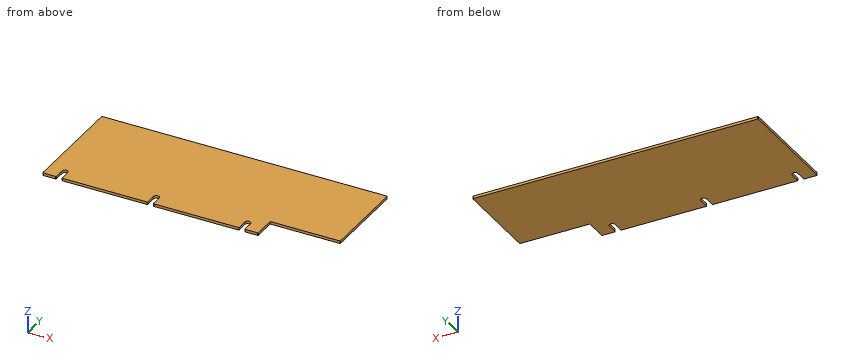
from build123d import *

# Parameters (mm, degrees)
PAD_DEPTH = 3


with BuildPart() as part:
    # Sketch → Pad (new body)
    with BuildSketch(Plane.XY):
        with BuildLine():
            Line((0, 126), (0, 1))
            ThreePointArc((0, 1), (0.292893, 0.292893), (1, 0))
            Line((1, 0), (14.748, 0))
            ThreePointArc((14.748, 0), (15.455107, 0.292893), (15.748, 1))
            Line((15.748, 12.7), (15.748, 1))
            ThreePointArc((22.352, 12.7), (19.05, 16.002), (15.748, 12.7))
            Line((22.352, 12.7), (22.352, 1))
            ThreePointArc((22.352, 1), (22.644893, 0.292893), (23.352, 0))
            Line((23.352, 0), (120.948, 0))
            ThreePointArc((120.948, 0), (121.655107, 0.292893), (121.948, 1))
            Line((121.948, 12.7), (121.948, 1))
            ThreePointArc((128.552, 12.7), (125.25, 16.002), (121.948, 12.7))
            Line((128.552, 12.7), (128.552, 1))
            ThreePointArc((128.552, 1), (128.844893, 0.292893), (129.552, 0))
            Line((129.552, 0), (227.148, 0))
            ThreePointArc((227.148, 0), (227.855107, 0.292893), (228.148, 1))
            Line((228.148, 12.7), (228.148, 1))
            ThreePointArc((234.752, 12.7), (231.45, 16.002), (228.148, 12.7))
            Line((234.752, 12.7), (234.752, 1))
            ThreePointArc((234.752, 1), (235.044893, 0.292893), (235.752, 0))
            Line((235.752, 0), (249.5, 0))
            ThreePointArc((249.5, 0), (250.207107, 0.292893), (250.5, 1))
            Line((250.5, 1), (250.5, 24.9))
            ThreePointArc((251.5, 25.9), (250.792893, 25.607107), (250.5, 24.9))
            Line((251.5, 25.9), (330.9999, 25.9))
            ThreePointArc((330.9999, 25.9), (331.707007, 26.192893), (331.9999, 26.9))
            Line((331.9999, 26.9), (331.9999, 126))
            ThreePointArc((331.9999, 126), (331.707007, 126.707107), (330.9999, 127))
            Line((330.9999, 127), (1, 127))
            ThreePointArc((1, 127), (0.292893, 126.707107), (0, 126))
        make_face()
    extrude(amount=PAD_DEPTH)


solid = part.part
Input: part model. Units: mm. Frame: model coordinates. Give positions to 0.01 mm unless a question says otherwise; leave off trailing zeros. Order: outer loops, then holes, each group sorted by start corner. A loop starts at its lowest first (then second) coordinate and runs counter-clockwise, first axis right, second up. Notation, with made-up numbers: (22.5, -25.75) - (62.5, -25.75) arc R9 cw to (62.5, -18.75) - close; hole circle Ø10 at (61, -17). An arc over 180 degrees is marked (long way). Answer as a JSON object with one key per item and string values. Group by question number.
Q1. Line query: probe 1 along X at (y, z) = (11.5, 2.6); probe 2 along Y at (x, z) = (297, 1); probe 3 along X at (y, z) = (19, 1.95). Output: solid intervals per line, ascending.
Q2. Cut plane B-B, the plane x = 19.05. Output: boundary loops of the cut face in (y, z).
Q3. First-contact query: pin 1 Ø0.9 at (y, z) = (6, 1.5) entering from +X; pin 2 Ø0.9 at (x, z) = (278.5, 1) entering from -Y. Flat tips, straight axial feed; report the tip coordinate or a pass-through.
Results:
{
 "1": {"probe 1": "0 to 15.75, 22.35 to 121.95, 128.55 to 228.15, 234.75 to 250.5", "probe 2": "25.9 to 127", "probe 3": "0 to 250.5"},
 "2": {"outline": "(16, 0) - (127, 0) - (127, 3) - (16, 3) - close"},
 "3": {"pin 1": "x = 250.5", "pin 2": "y = 25.9"}
}
